from build123d import *

# Parameters (mm, degrees)
F0_W      = 36
F0_H      = 10.7
F1_DEPTH  = 0.5
F2_W      = 24
F2_H      = 10.7
F3_DEPTH  = 6.2
F4_W      = 13
F4_H      = 6
F5_DEPTH  = 0.5
F6_W      = 6.8
F6_H      = 5.4
F7_DEPTH  = 8.7
F8_R      = 1.5
F9_DEPTH  = 0.5
F11_DEPTH = 0.5


# Not quite as in the source:
# - a pattern or mirror of a feature is missing from the dataset's text; its kind, count and spacing are read off the source's solid


with BuildPart() as f1:
    # F0 (on Top) → F1 (new body)
    with BuildSketch(Plane.XY):
        Rectangle(F0_W, F0_H)
    extrude(amount=F1_DEPTH)

    # F2 (on face) → F3 (join)
    with BuildSketch(Plane(origin=(0, 0, 0), x_dir=(1, 0, 0), z_dir=(0, 0, -1))):
        Rectangle(F2_W, F2_H)
    extrude(amount=F3_DEPTH)

    # F4 (on face) → F5 (cut)
    with BuildSketch(Plane.XY.offset(0.5)):
        Rectangle(F4_W, F4_H)
    extrude(amount=-F5_DEPTH, mode=Mode.SUBTRACT)

    # F6 (on face) → F7 (join)
    with BuildSketch(Plane.XY):
        with Locations((-3.1, 0)):
            Rectangle(F6_W, F6_H)
    extrude(amount=F7_DEPTH)

    # F8 (on face) → F9 (cut, through all)
    with BuildSketch(Plane.XY.offset(0.5)):
        with Locations((-16.1, 0)):
            Circle(F8_R)
        with Locations((16.1, 0)):
            Circle(F8_R)
    extrude(amount=-F9_DEPTH, mode=Mode.SUBTRACT)

    # F10 (on face) → F11 (cut, through all)
    with BuildSketch(Plane.XY.offset(0.5)):
        Polygon((-12, 3.85), (-12, 5.35), (-18, 5.35), (-18, 3.05), align=None)
        Polygon((-12, -3.85), (-18, -3.05), (-18, -5.35), (-12, -5.35), align=None)
    f11 = extrude(amount=-F11_DEPTH, mode=Mode.SUBTRACT)

    # F11_copies: F11 across plane
    add(f11.mirror(Plane(origin=(0, 0, 0), x_dir=(0, 0, 1), z_dir=(1, 0, 0))), mode=Mode.SUBTRACT)


solid = f1.part
Part model, mm, in its own coordinate system. A direction names the side the tool comes from. Coordinates: 2 decimals unless noted, no trailing zeros. Write each loop counter-clockwise with the first axis right and the second up, starting at its lowest first coordinate (ties: lowest second). Pieces come first, ordered by that corner, then holes. Notation, with made-up numbers: M 85.5,-39 L 133.5,-39 A15 cw 133.5,-24 Z; hole C 56.25,30 d4. An arc over 180 degrees is marked long. Return JSON: item names as keys, results as strings.
1. Pull direction X, two halves, no side cores. Call faces 1 (the face through (14.6, 0.07, 0.25)), 2 (the face through (-14, 0, 0)), 3 (the face through (-12, 0, -3)): pulls with the +X half, pulls with the -X half, needs draft (parallel to the pull), parting line crosses it, or undercut.
Determined:
{"face 1": "undercut", "face 2": "needs draft", "face 3": "pulls with the -X half"}
2. Saw through at C-C, the plane x = -3.5. Write the cut outline in (y, z), then the cut area to 3 significant figures.
Determined:
{"outline": "M -5.35,-6.2 L 5.35,-6.2 L 5.35,0.5 L 3,0.5 L 3,0 L 2.7,0 L 2.7,8.7 L -2.7,8.7 L -2.7,0 L -3,0 L -3,0.5 L -5.35,0.5 Z", "area": "116 mm²"}
3. Saw through at A-A, the plane x = 16.1. Write the cut outline in (y, z), then the cut area to 3 significant figures.
Determined:
{"outline": "M -3.3,0 L -1.5,0 L -1.5,0.5 L -3.3,0.5 Z; M 1.5,0 L 3.3,0 L 3.3,0.5 L 1.5,0.5 Z", "area": "1.80 mm²"}
4. Probe L1, parallel to X at y = -4, z = -3.25; L2, parallel to Z at x = 4.5, y = -2; L3, parallel to Z at x = 0, y = 4.75. List the from-to ranges inside material, lowest first.
Determined:
{"L1": "-12 to 12", "L2": "-6.2 to 0", "L3": "-6.2 to 0.5"}
5. 3-axis set-ups, long thin cutter, end or side, ignore diameter. For faces 4 (the face through (-6.5, 0, 5)), 5 (the face through (0, -5.35, -3)), 6 (the face through (14, 0, 0)): which of +Z, -Z, +X, -X, +Y, -Y reach the whole face in a straight line?
Determined:
{"face 4": "+Z, -X, +Y, -Y", "face 5": "+Z, -Z, +X, -X, -Y", "face 6": "-Z, +X, +Y, -Y"}
6. Flat gauge pins, fed straight in: pin 1 Ø3 at (x, y) = (-15.5, -0.5) entering from -Z; pin 2 Ø5.5 at (y, z) = (-2, -3) entering from +X; pin 3 Ø5 at (y, z) = (3, 5.5) entering from +X. Where does each tip first touch, or does it go through?
Determined:
{"pin 1": "z = 0", "pin 2": "x = 12", "pin 3": "x = 0.3"}
7. Saw through at D-D, the plane z = 4.5. Write the cut outline in (x, y).
Determined:
{"outline": "M -6.5,-2.7 L 0.3,-2.7 L 0.3,2.7 L -6.5,2.7 Z"}
8. Saw through at B-B, the plane y = -0.75. Write the cut outline in (x, z).
Determined:
{"outline": "M -18,0 L -17.4,0 L -17.4,0.5 L -18,0.5 Z; M -14.8,0 L -12,0 L -12,-6.2 L 12,-6.2 L 12,0 L 14.8,0 L 14.8,0.5 L 6.5,0.5 L 6.5,0 L 0.3,0 L 0.3,8.7 L -6.5,8.7 L -6.5,0.5 L -14.8,0.5 Z; M 17.4,0 L 18,0 L 18,0.5 L 17.4,0.5 Z"}
